```python
from build123d import *

# Parameters (mm, degrees)
SKETCH1_W           = 32
SKETCH1_H           = 12
BOSS_EXTRUDE1_DEPTH = 21.05
SKETCH2_W           = 15.014140453
SKETCH2_H           = 6
CUT_EXTRUDE1_DEPTH  = 46.435778853
SKETCH3_R           = 1.5
CUT_EXTRUDE2_DEPTH  = 6


with BuildPart() as part:
    # Sketch1 → Boss-Extrude1 (new, symmetric)
    with BuildSketch(Plane.XY):
        Rectangle(SKETCH1_W, SKETCH1_H)
    extrude(amount=BOSS_EXTRUDE1_DEPTH, both=True)

    # Sketch2 → Cut-Extrude1 (cut, through all)
    with BuildSketch(Plane.XY.offset(21.05)):
        with Locations((-0.007070226, -3)):
            Rectangle(SKETCH2_W, SKETCH2_H)
    extrude(amount=-CUT_EXTRUDE1_DEPTH, mode=Mode.SUBTRACT)

    # Sketch3 → Cut-Extrude2 (cut)
    with BuildSketch(Plane(origin=(0, 6, 0), x_dir=(1, 0, 0), z_dir=(0, 1, 0))):
        with Locations(Location((-12.5, 10, 0), (0, 0, 180))):
            Circle(SKETCH3_R)
        with Locations(Location((12.5, 10, 0), (0, 0, 180))):
            Circle(SKETCH3_R)
        with Locations(Location((12.5, -10, 0), (0, 0, 180))):
            Circle(SKETCH3_R)
        with Locations(Location((-12.5, -10, 0), (0, 0, 180))):
            Circle(SKETCH3_R)
    extrude(amount=-CUT_EXTRUDE2_DEPTH, mode=Mode.SUBTRACT)


solid = part.part
```
Source: CAD feature listing. Evaluate the final solid. Frame: model axes, mm. A direction names the side the tool comes from. Give positions to 0.01 mm unless a question says otherwise; leave off trailing zeros. Loops run counter-clockwise (first coordinate to the right, second up) from the corner with the lowest first, then second, coordinate; pieces in that order, holes last. Notation, with made-up numbers: (-7, 16) -> (1, 16) arc R10 ccw to (1, 34) -> close; hole circle Ø5 at (-1.75, 36). An arc over 180 degrees is marked (long way). Use a Markdown table: item, result. Add a question column.
(1) Section query B-B (z = 18.5). Output: boundary loops of the cut face in (x, y), then the cut area to 3 significant figures.
(2) Access query for faces 4 (the face through (12.825, 3.042, -11.464)), 5 (the face through (-7.514, -3, 0)), 6 (the face through (0, 1, 21.05)). Directions: +Z, -Z, +X, -X, +Y, -Y. A direction counts if a zero-diameter tool reaches every point of the face in a straight line with its end or side. Return the directions, or none.
(3) Section query D-D (y = 4). Output: boundary loops of the cut face in (x, z).
(4) Section query A-A (y = -2). Output: boundary loops of the cut face in (x, z), then the cut area to 3 significant figures.
(5) Ray query, line 1 (Z direction, x = -12.5, y = 1.6); line 2 (X direction, y = -5, z = 0); line 3 (X direction, y = 3.75, z = -9). Return the intervals inside material, ascending.
(6) Pull-direction query (X, two-part tool) for faces 1 (the face through (0, 1, -21.05)), 2 (the face through (13.7, 3, 9.1)), 3 (the face through (-16, 0, 0)); classes: +X half, -X half, draft (parallel to the pull), parting line (faces both ways), or undercut.
(7) Section query C-C (x = -12.5). Output: boundary loops of the cut face in (y, z), then the cut area to 3 significant figures.
(8) First-contact query: pin 1 Ø2.5 at (x, z) = (12.5, -10) entering from +Y; pin 2 Ø7.5 at (x, z) = (-2, 3.5) entering from -Y. Flat tips, straight axial feed; report the tip coordinate or a pass-through.
Checked values:
| question | item | result |
|---|---|---|
| 1 | outline | (-16, -6) -> (-7.51, -6) -> (-7.51, 0) -> (7.5, 0) -> (7.5, -6) -> (16, -6) -> (16, 6) -> (-16, 6) -> close |
| 1 | area | 294 mm^2 |
| 2 | face 4 | +Y |
| 2 | face 5 | +Z, -Z, -Y |
| 2 | face 6 | +Z, +X, -X, +Y, -Y |
| 3 | outline | (-16, -21.05) -> (16, -21.05) -> (16, 21.05) -> (-16, 21.05) -> close; hole circle Ø3 at (-12.5, -10); hole circle Ø3 at (-12.5, 10); hole circle Ø3 at (12.5, -10); hole circle Ø3 at (12.5, 10) |
| 4 | outline | (-16, -21.05) -> (-7.51, -21.05) -> (-7.51, 21.05) -> (-16, 21.05) -> close; (7.5, -21.05) -> (16, -21.05) -> (16, 21.05) -> (7.5, 21.05) -> close |
| 4 | area | 715 mm^2 |
| 5 | line 1 | -21.05 to -11.5, -8.5 to 8.5, 11.5 to 21.05 |
| 5 | line 2 | -16 to -7.51, 7.5 to 16 |
| 5 | line 3 | -16 to -13.62, -11.38 to 11.38, 13.62 to 16 |
| 6 | face 1 | draft |
| 6 | face 2 | undercut |
| 6 | face 3 | -X half |
| 7 | outline | (-6, -21.05) -> (6, -21.05) -> (6, -11.5) -> (0, -11.5) -> (0, -8.5) -> (6, -8.5) -> (6, 8.5) -> (0, 8.5) -> (0, 11.5) -> (6, 11.5) -> (6, 21.05) -> (-6, 21.05) -> close |
| 7 | area | 469 mm^2 |
| 8 | pin 1 | y = 0 |
| 8 | pin 2 | y = 0 |
